from build123d import *

# Parameters (mm, degrees)
BOSS_EXTRUDE1_DEPTH = 3
CUT_EXTRUDE1_REACH  = 245.11
SKETCH2_R           = 2.5


with BuildPart() as part:
    # Sketch1 → Boss-Extrude1 (new body)
    with BuildSketch(Plane.XY):
        with BuildLine():
            Line((-59.436088262, 179.5), (59.436088262, 179.5))
            ThreePointArc((59.436088262, 179.5), (73.578223886, 173.642135624), (79.436088262, 159.5))
            Line((79.436088262, 159.5), (79.436088262, 20))
            ThreePointArc((79.436088262, 20), (73.578223886, 5.857864376), (59.436088262, 0))
            Line((59.436088262, 0), (-153.931232863, 0))
            ThreePointArc((-153.931232863, 0), (-162.549941964, 4.928722701), (-162.672805625, 14.856429312))
            Line((-162.672805625, 14.856429312), (-76.919233785, 169.212858624))
            ThreePointArc((-76.919233785, 169.212858624), (-69.57864286, 176.737418201), (-59.436088262, 179.5))
        make_face()
    extrude(amount=BOSS_EXTRUDE1_DEPTH)

    # Sketch2 → Cut-Extrude1 (cut, up to next)
    with BuildSketch(Plane.XY.offset(3), mode=Mode.PRIVATE) as cut_extrude1_sk1:
        with Locations((-34.436088262, 169.5)):
            Circle(SKETCH2_R)
    cut_extrude1_tool1 = extrude(cut_extrude1_sk1.sketch, amount=-CUT_EXTRUDE1_REACH, mode=Mode.PRIVATE) & part.part
    # Sketch2 → Cut-Extrude1 (cut, up to next)
    with BuildSketch(Plane.XY.offset(3), mode=Mode.PRIVATE) as cut_extrude1_sk2:
        with Locations((34.433911738, 169.5)):
            Circle(SKETCH2_R)
    cut_extrude1_tool2 = extrude(cut_extrude1_sk2.sketch, amount=-CUT_EXTRUDE1_REACH, mode=Mode.PRIVATE) & part.part
    # Sketch2 → Cut-Extrude1 (cut, up to next)
    with BuildSketch(Plane.XY.offset(3), mode=Mode.PRIVATE) as cut_extrude1_sk3:
        with Locations((69.436088262, 134.5)):
            Circle(SKETCH2_R)
    cut_extrude1_tool3 = extrude(cut_extrude1_sk3.sketch, amount=-CUT_EXTRUDE1_REACH, mode=Mode.PRIVATE) & part.part
    # Sketch2 → Cut-Extrude1 (cut, up to next)
    with BuildSketch(Plane.XY.offset(3), mode=Mode.PRIVATE) as cut_extrude1_sk4:
        with Locations((69.436088262, 89.75)):
            Circle(SKETCH2_R)
    cut_extrude1_tool4 = extrude(cut_extrude1_sk4.sketch, amount=-CUT_EXTRUDE1_REACH, mode=Mode.PRIVATE) & part.part
    # Sketch2 → Cut-Extrude1 (cut, up to next)
    with BuildSketch(Plane.XY.offset(3), mode=Mode.PRIVATE) as cut_extrude1_sk5:
        with Locations((69.436088262, 45)):
            Circle(SKETCH2_R)
    cut_extrude1_tool5 = extrude(cut_extrude1_sk5.sketch, amount=-CUT_EXTRUDE1_REACH, mode=Mode.PRIVATE) & part.part
    # Sketch2 → Cut-Extrude1 (cut, up to next)
    with BuildSketch(Plane.XY.offset(3), mode=Mode.PRIVATE) as cut_extrude1_sk6:
        with Locations((24.436088262, 10)):
            Circle(SKETCH2_R)
    cut_extrude1_tool6 = extrude(cut_extrude1_sk6.sketch, amount=-CUT_EXTRUDE1_REACH, mode=Mode.PRIVATE) & part.part
    # Sketch2 → Cut-Extrude1 (cut, up to next)
    with BuildSketch(Plane.XY.offset(3), mode=Mode.PRIVATE) as cut_extrude1_sk7:
        with Locations((-47.243911738, 10)):
            Circle(SKETCH2_R)
    cut_extrude1_tool7 = extrude(cut_extrude1_sk7.sketch, amount=-CUT_EXTRUDE1_REACH, mode=Mode.PRIVATE) & part.part
    # Sketch2 → Cut-Extrude1 (cut, up to next)
    with BuildSketch(Plane.XY.offset(3), mode=Mode.PRIVATE) as cut_extrude1_sk8:
        with Locations((-118.923911738, 10)):
            Circle(SKETCH2_R)
    cut_extrude1_tool8 = extrude(cut_extrude1_sk8.sketch, amount=-CUT_EXTRUDE1_REACH, mode=Mode.PRIVATE) & part.part
    # Sketch2 → Cut-Extrude1 (cut, up to next)
    with BuildSketch(Plane.XY.offset(3), mode=Mode.PRIVATE) as cut_extrude1_sk9:
        with Locations((-134.505515616, 44.966291045)):
            Circle(SKETCH2_R)
    cut_extrude1_tool9 = extrude(cut_extrude1_sk9.sketch, amount=-CUT_EXTRUDE1_REACH, mode=Mode.PRIVATE) & part.part
    # Sketch2 → Cut-Extrude1 (cut, up to next)
    with BuildSketch(Plane.XY.offset(3), mode=Mode.PRIVATE) as cut_extrude1_sk10:
        with Locations((-87.602121323, 129.392400773)):
            Circle(SKETCH2_R)
    cut_extrude1_tool10 = extrude(cut_extrude1_sk10.sketch, amount=-CUT_EXTRUDE1_REACH, mode=Mode.PRIVATE) & part.part
    # Sketch2 → Cut-Extrude1 (cut, up to next)
    with BuildSketch(Plane.XY.offset(3), mode=Mode.PRIVATE) as cut_extrude1_sk11:
        with Locations((-111.05381847, 87.179345909)):
            Circle(SKETCH2_R)
    cut_extrude1_tool11 = extrude(cut_extrude1_sk11.sketch, amount=-CUT_EXTRUDE1_REACH, mode=Mode.PRIVATE) & part.part
    add(cut_extrude1_tool1.solids().sort_by_distance((-34.436088, 169.5, 3))[0], mode=Mode.SUBTRACT)
    add(cut_extrude1_tool2.solids().sort_by_distance((34.433912, 169.5, 3))[0], mode=Mode.SUBTRACT)
    add(cut_extrude1_tool3.solids().sort_by_distance((69.436088, 134.5, 3))[0], mode=Mode.SUBTRACT)
    add(cut_extrude1_tool4.solids().sort_by_distance((69.436088, 89.75, 3))[0], mode=Mode.SUBTRACT)
    add(cut_extrude1_tool5.solids().sort_by_distance((69.436088, 45, 3))[0], mode=Mode.SUBTRACT)
    add(cut_extrude1_tool6.solids().sort_by_distance((24.436088, 10, 3))[0], mode=Mode.SUBTRACT)
    add(cut_extrude1_tool7.solids().sort_by_distance((-47.243912, 10, 3))[0], mode=Mode.SUBTRACT)
    add(cut_extrude1_tool8.solids().sort_by_distance((-118.923912, 10, 3))[0], mode=Mode.SUBTRACT)
    add(cut_extrude1_tool9.solids().sort_by_distance((-134.505516, 44.966291, 3))[0], mode=Mode.SUBTRACT)
    add(cut_extrude1_tool10.solids().sort_by_distance((-87.602121, 129.392401, 3))[0], mode=Mode.SUBTRACT)
    add(cut_extrude1_tool11.solids().sort_by_distance((-111.053818, 87.179346, 3))[0], mode=Mode.SUBTRACT)


solid = part.part
Here's how the part is built. I have some questions about the finished solid (model axes, mm). Round coordinates to 2 decimals unless told otherwise and drop trailing zeros. Order: outer loops, then holes, each group sorted by start corner. A loop starts at its lowest first (then second) coordinate and runs counter-clockwise, first axis right, second up. Notation, with made-up numbers: (35.25, 30.5) -> (41.25, 30.5) arc R16 ccw to (41.25, 50.5) -> close; hole circle Ø9 at (57, 35.25). An arc over 180 degrees is marked (long way). Return JSON: item names as keys, results as strings.
Q1. If we section it at C-C on z = 2.3: Give the number of separate pieces and of enclosed holes in the cut face, plus the area to 3 significant figures.
Filled sheet:
{"separate pieces": "1", "enclosed holes": "11", "area": "35,500 mm^2"}
Q2. If we section it at A-A on y = 134.5: List the corners of the cut face in (x, z) for me.
Filled sheet:
{"outline": "(-96.2, 0) -> (66.94, 0) -> (66.94, 3) -> (-96.2, 3) -> close; (71.94, 0) -> (79.44, 0) -> (79.44, 3) -> (71.94, 3) -> close"}
Q3. For pin 1 Ø4.5 at (x, y) = (69.44, 45) entering from +Z; pin 2 Ø1.5 at (y, z) = (89.5, 1) entering from -X; pin 3 Ø1.5 at (x, z) = (-115.5, 0.5) entering from +Y, each with a flat end and sliding along its axis, tell me the tip position at first contact or that it passes through.
Filled sheet:
{"pin 1": "passes through", "pin 2": "stops at x = -121.62", "pin 3": "stops at y = 101.12"}
Q4. If we section it at B-B on y = 10: List the corners of the cut face in (x, z) for me.
Filled sheet:
{"outline": "(-163.93, 0) -> (-121.42, 0) -> (-121.42, 3) -> (-163.93, 3) -> close; (-116.42, 0) -> (-49.74, 0) -> (-49.74, 3) -> (-116.42, 3) -> close; (-44.74, 0) -> (21.94, 0) -> (21.94, 3) -> (-44.74, 3) -> close; (26.94, 0) -> (76.76, 0) -> (76.76, 3) -> (26.94, 3) -> close"}
Q5. If we mould it in two halves opening along Y, with no side actions, what happens to faces 1 (the flat face through (-14, 91, 3)), 2 (the cylindrical face through (-85.218, 130.143, 1.521)), 3 (the cylindrical face through (-34.76, 171.98, 1.52)), 4 (the cylindrical face through (73.73, 6.01, 1.48))? For each: released by +Y, released by -Y, zero draft, split by the parting line, or undercut.
Filled sheet:
{"face 1": "zero draft", "face 2": "undercut", "face 3": "undercut", "face 4": "released by -Y"}
Q6. If we section it at D-D on y = 106: List the corners of the cut face in (x, z) for me.
Filled sheet:
{"outline": "(-112.04, 0) -> (79.44, 0) -> (79.44, 3) -> (-112.04, 3) -> close"}
Q7. I need wall thicknesses on line 1 along X through (y, z) = (169.5, 2.35); line 2 along Y through (x, z) = (-134, 2); line 3 along X through (y, z) = (136, 2.6). Which ranges of each line are inside material? Lowest first, please. Write a range as from..to.
Filled sheet:
{"line 1": "x = -76.76..-36.94, -31.94..31.93, 36.93..76.76", "line 2": "y = 0..42.52, 47.41..66.47", "line 3": "x = -95.37..67.44, 71.44..79.44"}
